Input: part model. Units: mm. Frame: model coordinates. A direction names the side the tool comes from. Round coordinates to 2 decimals unless told otherwise and drop trailing zeros. Answer in a Markdown table with one row per item. Add a question column.
Q1. Ray query, L1, parallel to Y at x = 27, z = 0.5; L2, parallel to Y at x = 27.5, z = 1; L3, parallel to X at y = 2, z = 0. Return the intervals inside material, ascending. Write a range as from..to.
Q2. Section A-A, the plane x = 26.5. Give the number of separate pieces and of enclosed holes in the cut face, and give its area (3 significant figures).
Q3. Reachability of faces 1 (the face through (3.73, -26.83, -3.14)), 2 (the face through (21.23, 16.62, 0.04)) from +Z, -Z, +X, -X, +Y, -Y: full face, straight path, thin tool, end or side. Return the list, or none.
Q4. Mould query, pull axis X, two halves, no side actions, for faces 3 (the face through (-24.156, -21.341, 0.042)), 4 (the face through (7.09, 12.07, 0.04)), 5 (the face through (-12, -1, 3.5)). Classes: pulls with the +X half, pulls with the -X half, needs draft (parallel to the pull), parting line crosses it, or undercut.
Q5. Pin query (flat end, axial travel): pin 1 (1.5 mm diameter, centred on y = -26, z = 2, fed in from -X); pin 2 (4 mm diameter, centred on y = 5.5, z = -2, fed in from -X). Return the tip coordinate at first contact, or that it passes through.
```python
from build123d import *

# Parameters (mm, degrees)
F0_R     = 7.85
F0_R_2   = 11
F1_DEPTH = 3.5
F2_SIZE  = 0.5


with BuildPart() as f1:
    # F0 (on Top) → F1 (new body, symmetric)
    with BuildSketch(Plane.XY):
        with BuildLine():
            ThreePointArc((11.990417, -7.227026), (15.149203, -5.300815), (18.536452, -6.789025))
            ThreePointArc((18.536452, -6.789025), (30.738328, -10.185647), (37.845909, 0.297917))
            ThreePointArc((37.845909, 0.297917), (31.238527, 16.554265), (15.574074, 24.463201))
            ThreePointArc((15.574074, 24.463201), (21.25735, 16.476695), (18.717818, 7.009135))
            Line((18.717818, 7.009135), (18.536452, 6.789025))
            ThreePointArc((18.536452, 6.789025), (15.149203, 5.300815), (11.990417, 7.227026))
            ThreePointArc((11.990417, 7.227026), (7, 12.124356), (0.26358, 13.997519))
            ThreePointArc((0.26358, 13.997519), (-2.983961, 15.770002), (-3.388758, 19.447551))
            ThreePointArc((-3.388758, 19.447551), (-6.548135, 31.712997), (-19.180959, 32.62656))
            ThreePointArc((-19.180959, 32.62656), (-29.955678, 18.776225), (-28.972791, 1.255943))
            ThreePointArc((-28.972791, 1.255943), (-24.897911, 10.171058), (-15.428998, 12.705539))
            Line((-15.428998, 12.705539), (-15.147694, 12.658526))
            ThreePointArc((-15.147694, 12.658526), (-12.165242, 10.469187), (-12.253997, 6.770492))
            ThreePointArc((-12.253997, 6.770492), (-14, 0), (-12.253997, -6.770492))
            ThreePointArc((-12.253997, -6.770492), (-12.165242, -10.469187), (-15.147694, -12.658526))
            ThreePointArc((-15.147694, -12.658526), (-24.190193, -21.52735), (-18.664951, -32.924477))
            ThreePointArc((-18.664951, -32.924477), (-1.282849, -35.330491), (13.398717, -25.719144))
            ThreePointArc((13.398717, -25.719144), (3.640561, -26.647752), (-3.288821, -19.714673))
            Line((-3.288821, -19.714673), (-3.388758, -19.447551))
            ThreePointArc((-3.388758, -19.447551), (-2.983961, -15.770002), (0.26358, -13.997519))
            ThreePointArc((0.26358, -13.997519), (7, -12.124356), (11.990417, -7.227026))
        make_face()
        with BuildLine():
            ThreePointArc((4.290765, -29.959535), (-1.768845, -32.364165), (-8.267103, -32.887384))
            ThreePointArc((-8.267103, -32.887384), (-4.854938, -29.939011), (-2.936149, -25.858076))
            ThreePointArc((-2.936149, -25.858076), (0.377208, -28.437591), (4.290765, -29.959535))
        make_face(mode=Mode.SUBTRACT)
        with Locations((-13.5, -23.382686)):
            Circle(F0_R, mode=Mode.SUBTRACT)
        with BuildLine():
            ThreePointArc((-10.25149, -13.030407), (-9.535528, -11.916841), (-9.042029, -10.688391))
            ThreePointArc((-9.042029, -10.688391), (-7, -12.124356), (-4.735404, -13.174823))
            ThreePointArc((-4.735404, -13.174823), (-5.552523, -14.21643), (-6.158919, -15.393254))
            ThreePointArc((-6.158919, -15.393254), (-8.075, -13.98631), (-10.25149, -13.030407))
        make_face(mode=Mode.SUBTRACT)
        Circle(F0_R_2, mode=Mode.SUBTRACT)
        with BuildLine():
            ThreePointArc((-6.158919, 15.393254), (-5.552523, 14.21643), (-4.735404, 13.174823))
            ThreePointArc((-4.735404, 13.174823), (-7, 12.124356), (-9.042029, 10.688391))
            ThreePointArc((-9.042029, 10.688391), (-9.535528, 11.916841), (-10.25149, 13.030407))
            ThreePointArc((-10.25149, 13.030407), (-8.075, 13.98631), (-6.158919, 15.393254))
        make_face(mode=Mode.SUBTRACT)
        with BuildLine():
            ThreePointArc((-28.091101, 11.263856), (-27.143766, 17.713947), (-24.347759, 23.603213))
            ThreePointArc((-24.347759, 23.603213), (-23.500475, 19.174005), (-20.925676, 15.471818))
            ThreePointArc((-20.925676, 15.471818), (-24.816281, 13.892124), (-28.091101, 11.263856))
        make_face(mode=Mode.SUBTRACT)
        with Locations((-13.5, 23.382686)):
            Circle(F0_R, mode=Mode.SUBTRACT)
        with BuildLine():
            ThreePointArc((16.410408, -2.362847), (15.088051, -2.299589), (13.777433, -2.486431))
            ThreePointArc((13.777433, -2.486431), (14, 0), (13.777433, 2.486431))
            ThreePointArc((13.777433, 2.486431), (15.088051, 2.299589), (16.410408, 2.362847))
            ThreePointArc((16.410408, 2.362847), (16.15, 0), (16.410408, -2.362847))
        make_face(mode=Mode.SUBTRACT)
        with Locations((27, 0)):
            Circle(F0_R, mode=Mode.SUBTRACT)
        with BuildLine():
            ThreePointArc((23.800336, 18.695679), (28.912611, 14.650218), (32.614862, 9.284171))
            ThreePointArc((32.614862, 9.284171), (28.355413, 10.765006), (23.861825, 10.386258))
            ThreePointArc((23.861825, 10.386258), (24.439072, 14.545468), (23.800336, 18.695679))
        make_face(mode=Mode.SUBTRACT)
    extrude(amount=F1_DEPTH, both=True)

    # F2
    f2_edges = [f1.edges().sort_by_distance(p)[0] for p in [
        (7, -12.124356, -3.5),
        (-24.190193, -21.52735, -3.5),
        (3.640561, -26.647752, -3.5),
        (-24.897911, 10.171058, -3.5),
        (-29.955678, 18.776225, -3.5),
        (21.25735, 16.476695, -3.5),
        (21.25735, 16.476695, 3.5),
        (7, 12.124356, 3.5),
        (31.238527, 16.554265, 3.5),
        (3.640561, -26.647752, 3.5),
        (-1.282849, -35.330491, 3.5),
        (-24.897911, 10.171058, 3.5),
    ]]
    chamfer(f2_edges, length=F2_SIZE)


solid = f1.part
```
Answer block:
| question | item | result |
|---|---|---|
| 1 | L1 | -10.85..-7.85, 7.85..10.85, 16.46..20.23 |
| 1 | L2 | -10.84..-7.83, 7.83..10.84, 16.03..19.87 |
| 1 | L3 | -29.29..-28.96, -13.86..-10.82, 10.82..13.86, 16.34..19.41, 34.59..37.74 |
| 2 | separate pieces | 3 |
| 2 | enclosed holes | 0 |
| 2 | area | 67.3 mm^2 |
| 3 | face 1 | -Z |
| 3 | face 2 | +Z, -Z |
| 4 | face 3 | pulls with the -X half |
| 4 | face 4 | undercut |
| 4 | face 5 | needs draft |
| 5 | pin 1 | x = -24.19 |
| 5 | pin 2 | x = -30.8 |
